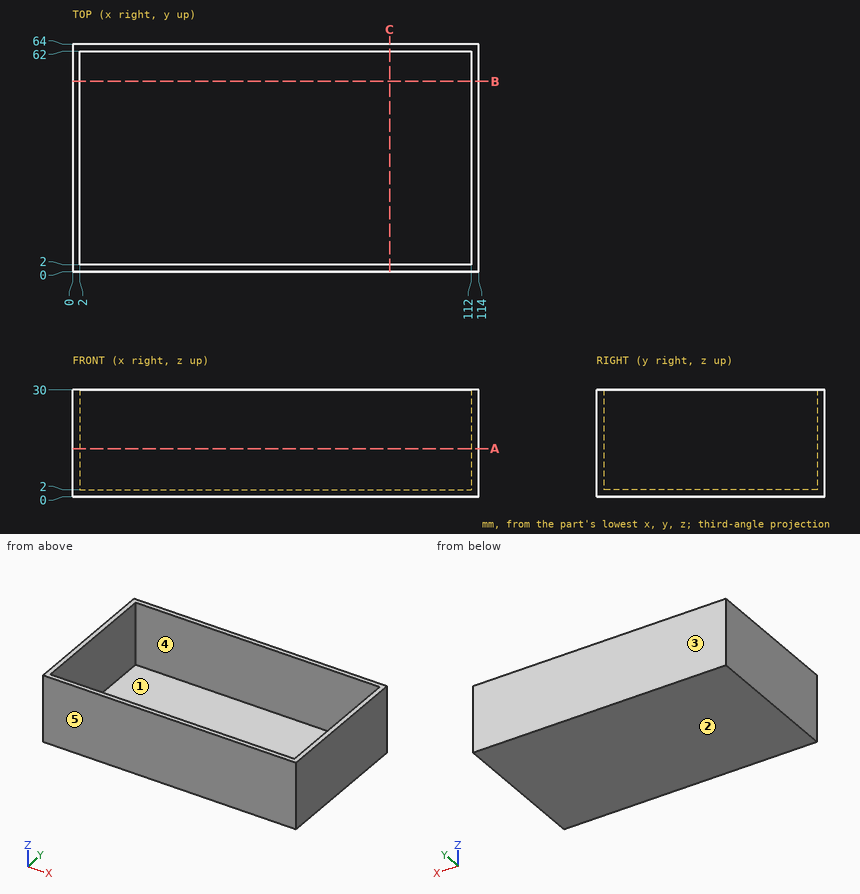
Verification items for this drawing (mm, ordinates from the low corner). A direction names the side the tool comes from. Give positions to 0.01 mm unless a question says otherwise; leave off trailing zeros. Write each loop counter-clockwise with the first axis right and the second up, starting at its lowest first coordinate (ties: lowest second). Pieces come first, ordered by that corner, then holes. Notation, with made-up numbers: M 23,51 L 73,51 A10 ccw 73,68 Z; hole C 50,82.5 d3. An arc over 180 degrees is marked long. Use one line per item in the form item = value.
(1) Section check B-B on y = 53.5. Record the boundary of the cut face in (x, z), plus the area to 3 significant figures.
Answer block:
outline = M 0,0 L 114,0 L 114,30 L 112,30 L 112,2 L 2,2 L 2,30 L 0,30 Z
area = 340 mm2
(2) Depth check by flat-ended pin: P1, Ø18, axis at x = 38.5, y = 40, coming from the +Z side. Enter the tip coordinate at first touch or a pass-through.
Answer block:
P1 = 2
(3) Material ranges on line 1 along Y through (x, z) = (6.5, 14); line 2 along X through (y, z) = (56, 3); line 3 along Z through (x, y) = (29.5, 18.5), recorded low to high.
Answer block:
line_1 = 0 to 2, 62 to 64
line_2 = 0 to 2, 112 to 114
line_3 = 0 to 2
(4) Section check C-C on x = 89. Record the boundary of the cut face in (y, z).
Answer block:
outline = M 0,0 L 64,0 L 64,30 L 62,30 L 62,2 L 2,2 L 2,30 L 0,30 Z
(5) Tool access check on the marked faces 4 and 5. Record the directions out of +Z, -Z, +X, -X, +Y, -Y that give a thin tool (end or side, any length) a straight path to the whole face; none if there is none.
Answer block:
face_4 = +Z
face_5 = +Z, -Z, +X, -X, -Y
(6) Section check A-A on z = 13.5. Record the boundary of the cut face in (x, y).
Answer block:
outline = M 0,0 L 114,0 L 114,64 L 0,64 Z; hole M 2,2 L 112,2 L 112,62 L 2,62 Z
(7) Draft check along Y on the marked faces 1, 2 and 3. Enter one of: pulls with the +Y half, pulls with the -Y half, needs draft (parallel to the pull), parting line crosses it, or undercut.
Answer block:
face_1 = undercut
face_2 = needs draft
face_3 = pulls with the +Y half
